```python
from build123d import *

# Parameters (mm, degrees)
SKETCH1_W           = 13.208
SKETCH1_H           = 13.208
BOSS_EXTRUDE1_DEPTH = 190.5
SKETCH3_W           = 213.36
SKETCH3_H           = 88.9
SKETCH3_H_2         = 76.2
CUT_EXTRUDE2_DEPTH  = 304.8


with BuildPart() as part:
    # Sketch1 → Boss-Extrude1 (new body)
    with BuildSketch(Plane(origin=(0, 0, 0), x_dir=(1, 0, 0), z_dir=(0, 1, 0))):
        Polygon((106.68, 120.142), (0, 120.142), (0, 0), (106.68, 0), (106.68, 106.934), align=None)
        with Locations((113.284, 113.538)):
            Rectangle(SKETCH1_W, SKETCH1_H)
        Polygon((106.68, 0), (0, 0), (0, -120.142), (106.68, -120.142), (106.68, -106.934), align=None)
        Polygon((0, -120.142), (0, 0), (-106.68, 0), (-106.68, -106.934), (-106.68, -120.142), align=None)
        with Locations((-113.284, -113.538)):
            Rectangle(SKETCH1_W, SKETCH1_H)
        Polygon((0, 0), (0, 120.142), (-106.68, 120.142), (-106.68, 106.934), (-106.68, 0), align=None)
        with Locations((-113.284, 113.538)):
            Rectangle(SKETCH1_W, SKETCH1_H)
        with Locations((113.284, -113.538)):
            Rectangle(SKETCH1_W, SKETCH1_H)
    extrude(amount=BOSS_EXTRUDE1_DEPTH)

    # Sketch3 → Cut-Extrude2 (cut)
    with BuildSketch(Plane.XY.offset(120.142)):
        with Locations((0, 57.15)):
            Rectangle(SKETCH3_W, SKETCH3_H)
        with Locations((0, 152.4)):
            Rectangle(SKETCH3_W, SKETCH3_H_2)
    extrude(amount=-CUT_EXTRUDE2_DEPTH, mode=Mode.SUBTRACT)


solid = part.part
```
Geometry check sheet. Reference: the model listing, model coordinates, mm. A direction names the side the tool comes from. Give positions to 0.01 mm unless a question says otherwise; leave off trailing zeros. Loops run counter-clockwise (first coordinate to the right, second up) from the corner with the lowest first, then second, coordinate; pieces in that order, holes last. Notation, with made-up numbers: M 44,19 L 82,19 A19 ccw 82,30 Z; hole C 28.25,57 d11. An arc over 180 degrees is marked long. Answer as CSV lines item,"result".
Item 1: Cross-section at A-A on z = -13. Record the cut outline in (x, y), and give its area (3 significant figures).
Values:
outline,"M -106.68,0 L 106.68,0 L 106.68,12.7 L -106.68,12.7 Z; M -106.68,101.6 L 106.68,101.6 L 106.68,114.3 L -106.68,114.3 Z"
area,"5,420 mm²"
Item 2: Cross-section at C-C on y = 42. Record the cut outline in (x, z).
Values:
outline,"M -119.89,-120.14 L -106.68,-120.14 L -106.68,-106.93 L -119.89,-106.93 Z; M -119.89,106.93 L -106.68,106.93 L -106.68,120.14 L -119.89,120.14 Z; M 106.68,-120.14 L 119.89,-120.14 L 119.89,-106.93 L 106.68,-106.93 Z; M 106.68,106.93 L 119.89,106.93 L 119.89,120.14 L 106.68,120.14 Z"
Item 3: Cross-section at B-B on x = -69. Record the cut outline in (y, z).
Values:
outline,"M 0,-120.14 L 12.7,-120.14 L 12.7,120.14 L 0,120.14 Z; M 101.6,-120.14 L 114.3,-120.14 L 114.3,120.14 L 101.6,120.14 Z"
Item 4: Cross-section at D-D on y = 108. Record the cut outline in (x, z), and give its area (3 significant figures).
Values:
outline,"M -119.89,-120.14 L 119.89,-120.14 L 119.89,-106.93 L 106.68,-106.93 L 106.68,106.93 L 119.89,106.93 L 119.89,120.14 L -119.89,120.14 L -119.89,106.93 L -106.68,106.93 L -106.68,-106.93 L -119.89,-106.93 Z"
area,"52,000 mm²"
Item 5: Material ranges on line 1 (Y direction, x = -49, z = 1.5); line 2 (X direction, y = 96, z = 110); line 3 (X direction, y = 112, z = -86), recorded low to high.
Values:
line 1,"y = 0 to 12.7, 101.6 to 114.3"
line 2,"x = -119.89 to -106.68, 106.68 to 119.89"
line 3,"x = -106.68 to 106.68"
Item 6: Access from +Z, -Z, +X, -X, +Y, -Y to the whole of each face (thin tool, end or side, straight path). Record for faces 5 (the flat face through (-106.68, 57, 114)), 6 (the flat face through (106.68, 6, 1)), 7 (the flat face through (-119.888, 94, -113)), 8 (the flat face through (106.68, 152, -113)).
Values:
face 5,"+Z, -Z"
face 6,"+X, +Y, -Y"
face 7,"+Z, -Z, -X, +Y, -Y"
face 8,"+Z, -Z, +Y"
Item 7: Depth check by flat-ended pin: P1, Ø10, axis at y = 5, z = -26, coming from the -X side; P2, Ø1, axis at x = -64.5, z = 5.5, coming from the -Y side; P3, Ø14, axis at y = 109, z = 38.5, coming from the +X side. Enter the tip coordinate at first touch or a pass-through.
Values:
P1,"stops at x = -106.68"
P2,"stops at y = 0"
P3,"stops at x = 106.68"
Item 8: Release check for a two-part mould opening along Z. For faces 1 (the flat face through (-106.68, 6, -1)), 2 (the flat face through (106.68, 57, -113)), 3 (the flat face through (-27, 102, 120.142)), 4 (the flat face through (113, 94, -106.934)) record: pulls with the +Z half, pulls with the -Z half, needs draft (parallel to the pull), parting line crosses it, or undercut.
Values:
face 1,"undercut"
face 2,"needs draft"
face 3,"pulls with the +Z half"
face 4,"undercut"
